from build123d import *

# Parameters (mm, degrees)
FILLET1_R = 0.4


with BuildPart() as part:
    # Sketch1 → Revolve1 (revolve)
    with BuildSketch(Plane(origin=(0, 0, 0), x_dir=(0, 0, -1), z_dir=(1, 0, 0))):
        Polygon((0, 0), (-12.5, 0), (-12.5, 3), (-9.8, 3), (-9.8, 8.7), (-9, 13.2), (-5, 13.2), (-5, 2.8), (0, 2.8), align=None)
    revolve(axis=Axis((0, 0, 0), (0, 1, 0)))

    # Fillet1
    fillet1_edges = [part.edges().sort_by_distance(p)[0] for p in [
        (0, 0, -12.5),
    ]]
    fillet(fillet1_edges, radius=FILLET1_R)


solid = part.part
Model file for the job. Use its own axes, mm. A direction names the side the tool comes from. Coordinates: 2 decimals unless noted, no trailing zeros. Write each loop counter-clockwise with the first axis right and the second up, starting at its lowest first coordinate (ties: lowest second). Pieces come first, ordered by that corner, then holes. Notation, with made-up numbers: (-10, -1.5) -> (-5, -1.5) arc R25 ccw to (-5, 24.5) -> close; hole circle Ø10 at (-18, 51.25). An arc over 180 degrees is marked (long way). One line per item, written item: value. Start each with the question number.
1) Which spindle directions (+Z, -Z, +X, -X, +Y, -Y) get a long thin tool onto all of the face, cutting with end or side? Do faces 4 (the face through (0, 0, 0)), 5 (the face through (-4.88, 7.93, -1.08)). Say none if no direction does.
2) Pull direction Z, two halves, no side cores. Call faces 1 (the face through (0, 2.8, 0)), 2 (the face through (-8.3, 3, 5.5)), 3 (the face through (3.755, 1.718, 11.923)): +Z half, -Z half, draft (parallel to the pull), parting line (faces both ways), or undercut.
3) Flat gauge pins, fed straight in: pin 1 Ø1 at (x, y) = (-5.5, 12) entering from +Z; pin 2 Ø6 at (y, z) = (10.5, -9.5) entering from +X; pin 3 Ø4 at (x, y) = (5.5, 8) entering from -Z. Where does each tip first touch, or does it go through?
4) Slice it at D-D on y = 10. Write the cut outline in (x, z), then the cut area to 3 significant figures.
5) Slice it at C-C on y = 8.25. Write the cut outline in (x, z).
6) Slice it at A-A on z = 0. Write the cut outline in (x, y), then the cut area to 3 significant figures.
7) Slice it at B-B on x = 0. Write the cut outline in (y, z), then the cut area to 3 significant figures.
8) Probe probe 1 along X at (y, z) = (5.5, 0); probe 2 along Y at (x, z) = (1.5, -4.5); probe 3 along Z at (x, y) = (3.25, 6.25). List the from-to ranges inside material, lowest first.
Answers follow:
1. face 4: +Z, -Z, +X, -X, -Y
1. face 5: +Y
2. face 1: undercut
2. face 2: draft
2. face 3: parting line
3. pin 1: z = 7.76
3. pin 2: x = 6.99
3. pin 3: z = -9.15
4. outline: circle Ø19.14 at (0, 0); hole circle Ø10 at (0, 0)
4. area: 209 mm2
5. outline: circle Ø19.6 at (0, 0); hole circle Ø10 at (0, 0)
6. outline: (-12.5, 0.4) arc R0.4 ccw to (-12.1, 0) -> (12.1, 0) arc R0.4 ccw to (12.5, 0.4) -> (12.5, 3) -> (9.8, 3) -> (9.8, 8.7) -> (9, 13.2) -> (5, 13.2) -> (5, 2.8) -> (-5, 2.8) -> (-5, 13.2) -> (-9, 13.2) -> (-9.8, 8.7) -> (-9.8, 3) -> (-12.5, 3) -> close
6. area: 167 mm2
7. outline: (0, -12.1) arc R0.4 ccw to (0.4, -12.5) -> (3, -12.5) -> (3, -9.8) -> (8.7, -9.8) -> (13.2, -9) -> (13.2, -5) -> (2.8, -5) -> (2.8, 5) -> (13.2, 5) -> (13.2, 9) -> (8.7, 9.8) -> (3, 9.8) -> (3, 12.5) -> (0.4, 12.5) arc R0.4 ccw to (0, 12.1) -> close
7. area: 167 mm2
8. probe 1: -9.8 to -5, 5 to 9.8
8. probe 2: 0 to 2.8
8. probe 3: -9.25 to -3.8, 3.8 to 9.25
